Answer from the drawing. Dimensions are ordinates in mm from the lowest x, y and z of the part. A direction names the side the tool comes from. Round coordinates to 2 decimals unless told otherwise and drop trailing zeros. Loops run counter-clockwise (first coordinate to the right, second up) from the corner with the lowest first, then second, coordinate; pieces in that order, holes last. Notation, with made-up numbers: (65.25, 68) - (78.25, 68) arc R18 ccw to (78.25, 82) - close; hole circle Ø6 at (63.5, -34). An arc over 180 degrees is marked (long way). Answer as CSV lines item,"result". Start each with the question number.
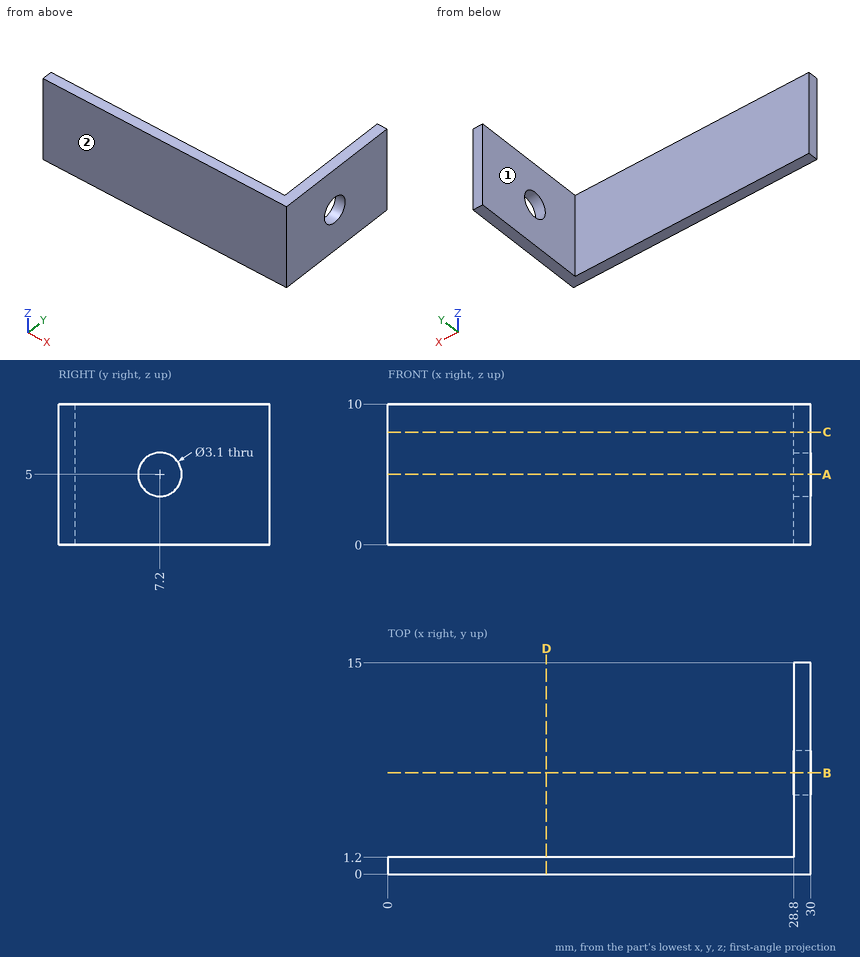
Item 1: Find the intervals of material crossed by L1, parallel to Z at x = 29.3, y = 7.2; L2, parallel to Y at x = 19.5, z = 2.75; L3, parallel to X at y = 10.75, z = 7.75, in increasing order.
Item 2: Section B-B, the plane y = 7.2 is taken. Give the vertices of the cut face in (x, z), and give its area (3 significant figures).
Item 3: Section C-C, the plane z = 8 is taken. Give the vertices of the cut face in (x, y).
Item 4: Section D-D, the plane x = 11.25 is taken. Give the vertices of the cut face in (y, z), and give its area (3 significant figures).
Item 5: Which of the six approach directions +Z, -Z, +X, -X, +Y, -Y give full straight-line access (tool end or side, diameter ignored) to the marked faces 1 and 2?
Item 6: Section A-A, the plane z = 5 is taken. Give the vertices of the cut face in (x, y), and give its area (3 significant figures).
Item 7: Flat-ended cylindrical pins translate along their axes: pin 1 Ø3 at (x, z) = (10.5, 4.5) entering from +Y; pin 2 Ø3 at (y, z) = (9, 3) entering from -X; pin 3 Ø1.5 at (x, z) = (10.5, 2.5) entering from -Y. Find the tip coordinate at first contact, or state that the pin passes through.
Answer:
1,L1,"z = 0 to 3.45, 6.55 to 10"
1,L2,"y = 0 to 1.2"
1,L3,"x = 28.8 to 30"
2,outline,"(28.8, 0) - (30, 0) - (30, 3.45) - (28.8, 3.45) - close; (28.8, 6.55) - (30, 6.55) - (30, 10) - (28.8, 10) - close"
2,area,"8.28 mm²"
3,outline,"(0, 0) - (30, 0) - (30, 15) - (28.8, 15) - (28.8, 1.2) - (0, 1.2) - close"
4,outline,"(0, 0) - (1.2, 0) - (1.2, 10) - (0, 10) - close"
4,area,"12.0 mm²"
5,face 1,"+Z, -Z, -X, +Y"
5,face 2,"+Z, -Z, +X, -X, -Y"
6,outline,"(0, 0) - (30, 0) - (30, 5.65) - (28.8, 5.65) - (28.8, 1.2) - (0, 1.2) - close; (28.8, 8.75) - (30, 8.75) - (30, 15) - (28.8, 15) - close"
6,area,"48.8 mm²"
7,pin 1,"stops at y = 1.2"
7,pin 2,"stops at x = 28.8"
7,pin 3,"stops at y = 0"
